Here's how the part is built. I have some questions about the finished solid (model axes, mm). Face numbers are marked on the shaded views. A direction names the side the tool comes from. Give positions to 0.01 mm unless a question says otherwise; leave off trailing zeros. Loops run counter-clockwise (first coordinate to the right, second up) from the corner with the lowest first, then second, coordinate; pieces in that order, holes last. Notation, with made-up numbers: (75, -25.75) - (117, -25.75) arc R28 cw to (117, -6.75) - close; hole circle Ø5 at (52.5, 26.5). An arc over 180 degrees is marked (long way). Use one line per item in the form item = value.
from build123d import *

# Parameters (mm, degrees)
F0_W     = 38.1
F0_H     = 38.1
F0_R     = 10.541
F1_DEPTH = 6.35
F0_R_2   = 7.9375
F2_DEPTH = 6.35
F3_D     = 4.4958
F4_D     = 4.4958
F5_D     = 4.4958
F6_D     = 4.4958
F7_DEPTH = 4.365625


with BuildPart() as f1:
    # F0 (on Top) → F1 (new body)
    with BuildSketch(Plane.XY):
        Rectangle(F0_W, F0_H)
        Circle(F0_R, mode=Mode.SUBTRACT)
    extrude(amount=F1_DEPTH)

    # F0 (on Top) → F2 (join)
    with BuildSketch(Plane.XY):
        Rectangle(F0_W, F0_H)
        Circle(F0_R, mode=Mode.SUBTRACT)
        Circle(F0_R)
        Circle(F0_R_2, mode=Mode.SUBTRACT)
    extrude(amount=F2_DEPTH)

    # F3 (through all)
    with Locations(Plane(origin=(0, 0, 0), x_dir=(1, 0, 0), z_dir=(0, 0, -1))):
        with Locations((-13.4747, 13.4747)):
            Hole(F3_D / 2)

    # F4 (through all)
    with Locations(Plane(origin=(0, 0, 0), x_dir=(1, 0, 0), z_dir=(0, 0, -1))):
        with Locations((-13.4747, -13.4747)):
            Hole(F4_D / 2)

    # F5 (through all)
    with Locations(Plane(origin=(0, 0, 0), x_dir=(1, 0, 0), z_dir=(0, 0, -1))):
        with Locations((13.4747, -13.4747)):
            Hole(F5_D / 2)

    # F6 (through all)
    with Locations(Plane(origin=(0, 0, 0), x_dir=(1, 0, 0), z_dir=(0, 0, -1))):
        with Locations((13.4747, 13.4747)):
            Hole(F6_D / 2)

    # F0 (on Top) → F7 (cut)
    with BuildSketch(Plane.XY):
        Circle(F0_R)
        Circle(F0_R_2, mode=Mode.SUBTRACT)
    extrude(amount=F7_DEPTH, mode=Mode.SUBTRACT)


solid = f1.part
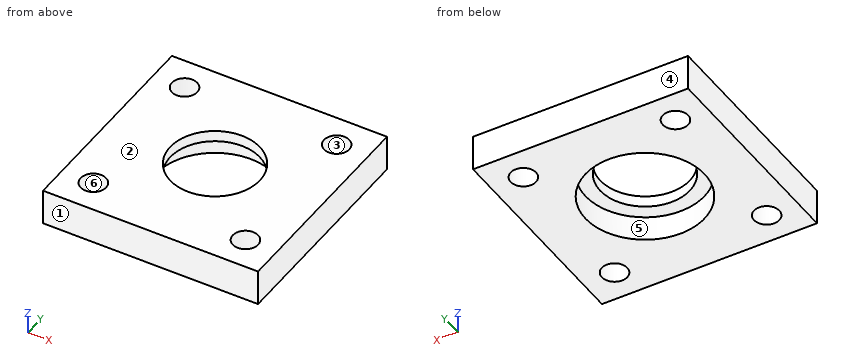
(1) If I drill on probe 1 along Y at (x, z) = (-13.5, 6); probe 2 along Y at (x, z) = (0, 2.7); probe 3 along Y at (x, z) = (0, 5.3), over which ranges is the centre line in solid material (lowest first)?
Geometry says:
probe_1 = -19.05 to -15.72, -11.23 to 11.23, 15.72 to 19.05
probe_2 = -19.05 to -10.54, 10.54 to 19.05
probe_3 = -19.05 to -7.94, 7.94 to 19.05
(2) If we section it at C-C (x = -13): List the corners of the cut face in (y, z) for me.
Geometry says:
outline = (-19.05, 0) - (-15.67, 0) - (-15.67, 6.35) - (-19.05, 6.35) - close; (-11.28, 0) - (11.28, 0) - (11.28, 6.35) - (-11.28, 6.35) - close; (15.67, 0) - (19.05, 0) - (19.05, 6.35) - (15.67, 6.35) - close
(3) If we section it at D-D (y = -12): List the corners of the cut face in (x, z) for me.
Geometry says:
outline = (-19.05, 0) - (-15.17, 0) - (-15.17, 6.35) - (-19.05, 6.35) - close; (-11.78, 0) - (11.78, 0) - (11.78, 6.35) - (-11.78, 6.35) - close; (15.17, 0) - (19.05, 0) - (19.05, 6.35) - (15.17, 6.35) - close
(4) For the marked faces 5 and 6, which set-ups out of +Z, -Z, +X, -X, +Y, -Y let a thin tool reach every point of the face, with its end or its side?
Geometry says:
face_5 = -Z
face_6 = +Z, -Z
(5) Thinking about a two-plate mould opening in Y: for the marked faces 1, 2, 3 and 4, which applies, pulls with the +Y half, pulls with the -Y half, needs draft (parallel to the pull), parting line crosses it, or undercut?
Geometry says:
face_1 = pulls with the -Y half
face_2 = needs draft
face_3 = undercut
face_4 = pulls with the +Y half
(6) If we section it at A-A (y = 0): List the corners of the cut face in (x, z) for me, plus the area to 3 significant figures.
Geometry says:
outline = (-19.05, 0) - (-10.54, 0) - (-10.54, 4.37) - (-7.94, 4.37) - (-7.94, 6.35) - (-19.05, 6.35) - close; (7.94, 4.37) - (10.54, 4.37) - (10.54, 0) - (19.05, 0) - (19.05, 6.35) - (7.94, 6.35) - close
area = 118 mm²
(7) For P1, Ø2, axis at x = 7.5, y = -4, coming from the -Z side; P2, Ø3.5, axis at x = 13.47, y = 13.47, coming from the -Z side, each with a flat end and sliding along its axis, tell me the tip position at first contact or that it passes through.
Geometry says:
P1 = 4.37
P2 = through
